Study the drawing (mm; zero at the part's minimum x, y, z) and answer. A direction names the side the tool comes from. Coordinates: 2 decimals unless noted, no trailing zeros. Loops run counter-clockwise (first coordinate to the right, second up) from the corner with the lowest first, then second, coordinate; pieces in that order, holes last. Notation, with made-up numbers: (58.5, 67) - (116.5, 67) arc R22 ccw to (116.5, 90) - close; hole circle Ø9 at (25.5, 69). An arc over 180 degrees is marked (long way). Use one line per item in the form item = value.
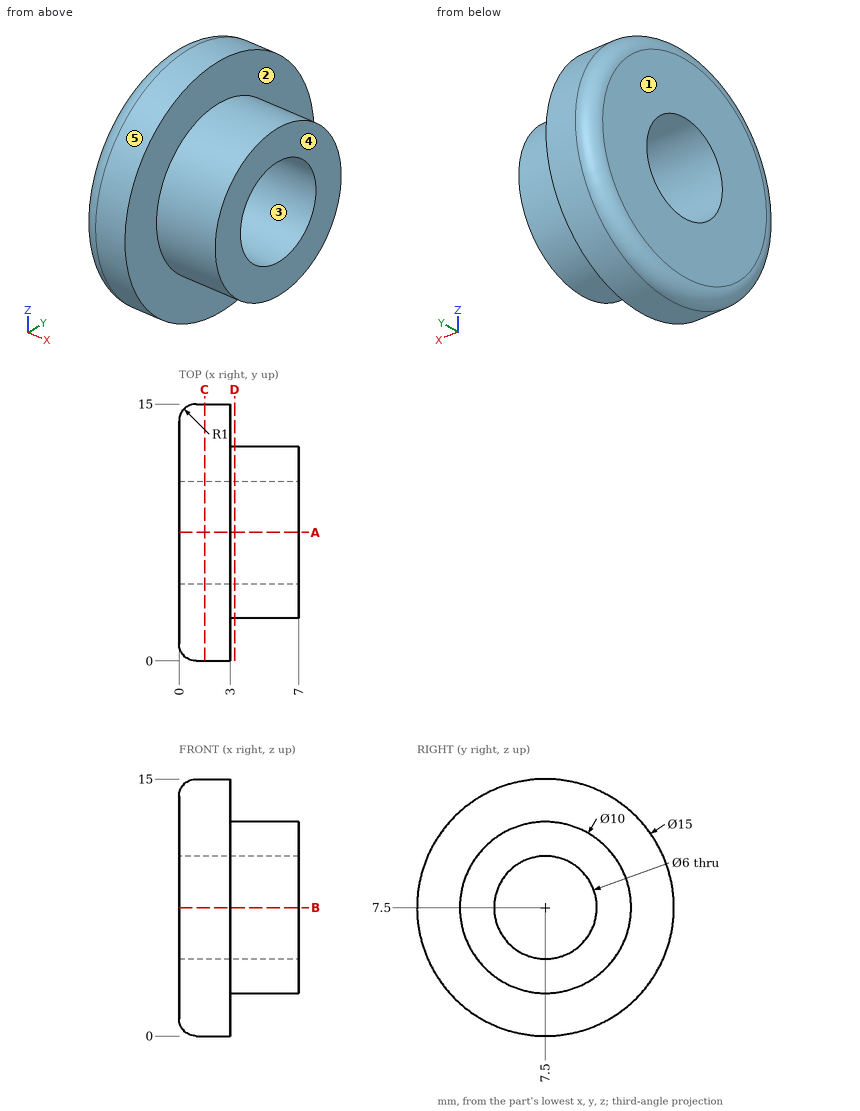
Item 1: This flat-tipped pin is pushed along its axis until it touches: P1, Ø2, axis at x = 6, y = 12.5, coming from the -Z side. Where does it stop, or does it pass through?
Results below:
P1 = 4.5
Item 2: Find the intervals of material crossed by L1, parallel to Y at x = 1.75, z = 7.5; L2, parallel to Y at x = 4.5, z = 7.5; L3, parallel to X at y = 4, z = 12.5, in increasing order.
Results below:
L1 = 0 to 4.5, 10.5 to 15
L2 = 2.5 to 4.5, 10.5 to 12.5
L3 = 0 to 3
Item 3: The part is cut by section C-C on x = 1.5. Give the vertices of the cut face in (y, z).
Results below:
outline = circle Ø15 at (7.5, 7.5); hole circle Ø6 at (7.5, 7.5)
Item 4: The part is cut by section A-A on y = 7.5. Give the vertices of the cut face in (x, z), plus the area to 3 significant figures.
Results below:
outline = (0, 1) arc R1 ccw to (1, 0) - (3, 0) - (3, 2.5) - (7, 2.5) - (7, 4.5) - (0, 4.5) - close; (0, 10.5) - (7, 10.5) - (7, 12.5) - (3, 12.5) - (3, 15) - (1, 15) arc R1 ccw to (0, 14) - close
area = 42.6 mm²
Item 5: The part is cut by section D-D on x = 3.25. Give the vertices of the cut face in (y, z).
Results below:
outline = circle Ø10 at (7.5, 7.5); hole circle Ø6 at (7.5, 7.5)
Item 6: Which of the six approach directions +Z, -Z, +X, -X, +Y, -Y give full straight-line access (tool end or side, diameter ignored) to the marked faces 1 and 2?
Results below:
face_1 = +Z, -Z, -X, +Y, -Y
face_2 = +X
Item 7: For a pull along Y with two mould halves and no side action, classify the marked faces 3, 4 and 5 as +Y half, -Y half, draft (parallel to the pull), parting line (faces both ways), or undercut.
Results below:
face_3 = undercut
face_4 = draft
face_5 = parting line
